The drawing under review shows one solid part. Ordinate dimensions are in mm from its lowest x, y, z. A direction names the side the tool comes from. Round coordinates to 2 decimals unless told otherwise and drop trailing zeros. Write each loop counter-clockwise with the first axis right and the second up, starting at its lowest first coordinate (ties: lowest second). Pieces come first, ordered by that corner, then holes. Notation, with made-up numbers: (82, -34.75) -> (140, -34.75) arc R31 ccw to (140, -0.75) -> close; hole circle Ø1 at (15, 55.25). An arc over 180 degrees is marked (long way). Write item = value, one per line. Start each with the question number.
Item 1: Add section D-D, the plane y = 3.85. State the section outline as (x, z) points, then the cut area to 3 significant figures.
Item 2: Machinability: for the marked faces 1 and 2, which of the approach directions +Z, -Z, +X, -X, +Y, -Y give a long, thin tool a straight path to every point of the face, cutting with its end or side? Answer none if there is none.
Item 3: Add section B-B, the plane y = 0.9. State the section outline as (x, z) points.
Item 4: Add section C-C, the plane z = 4. State the section outline as (x, y) points, then the cut area to 4 significant figures.
Item 5: Add section A-A, the plane x = 20. State the section outline as (y, z) points.
Item 6: Mouldability with a two-part tool opening along Z and no side actions: class the marked faces 3, 4, 5 and 6 as released by +Z, released by -Z, zero draft, split by the parting line, or undercut.
Item 7: To check wall thickness, follow L1, parallel to X at y = 0.7, z = 2.75; L2, parallel to Z at x = 2.75, y = 1.3; L3, parallel to Y at x = 12.25, z = 1.5. State the ranges of each line that lie inside material, in increasing order.
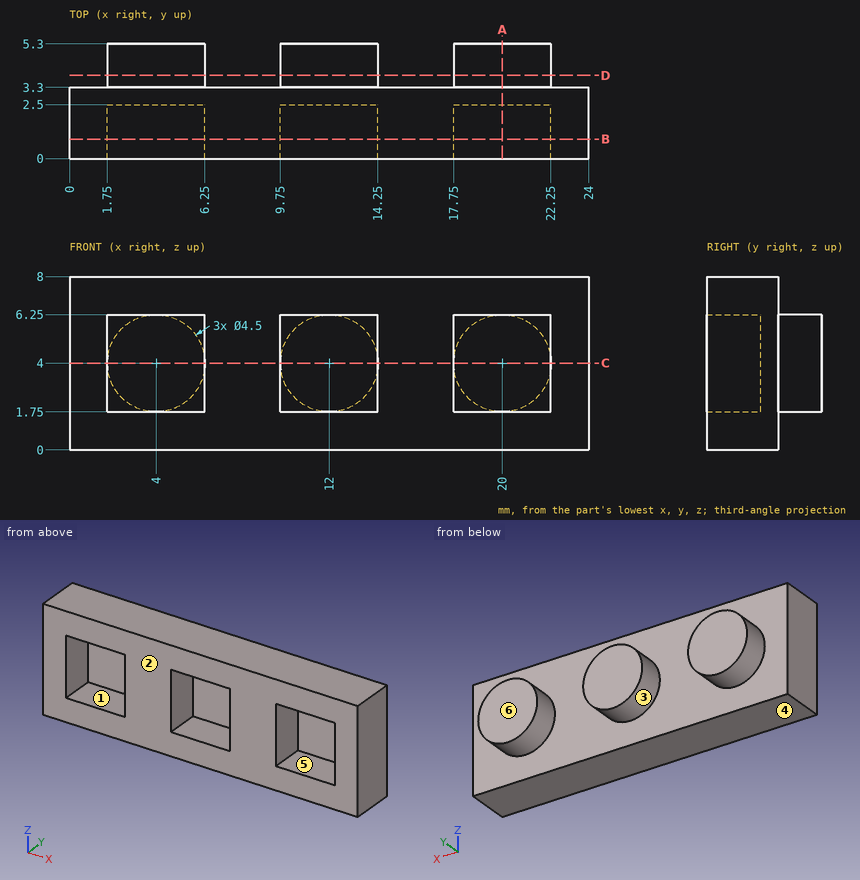
Result set:
q1.outline = circle Ø4.5 at (4, 4); circle Ø4.5 at (12, 4); circle Ø4.5 at (20, 4)
q1.area = 47.7 mm²
q2.face_1 = -Y
q2.face_2 = +Z, -Z, +X, -X, -Y
q3.outline = (0, 0) -> (24, 0) -> (24, 8) -> (0, 8) -> close; hole (1.75, 1.75) -> (6.25, 1.75) -> (6.25, 6.25) -> (1.75, 6.25) -> close; hole (9.75, 1.75) -> (14.25, 1.75) -> (14.25, 6.25) -> (9.75, 6.25) -> close; hole (17.75, 1.75) -> (22.25, 1.75) -> (22.25, 6.25) -> (17.75, 6.25) -> close
q4.outline = (0, 0) -> (1.75, 0) -> (1.75, 2.5) -> (6.25, 2.5) -> (6.25, 0) -> (9.75, 0) -> (9.75, 2.5) -> (14.25, 2.5) -> (14.25, 0) -> (17.75, 0) -> (17.75, 2.5) -> (22.25, 2.5) -> (22.25, 0) -> (24, 0) -> (24, 3.3) -> (22.25, 3.3) -> (22.25, 5.3) -> (17.75, 5.3) -> (17.75, 3.3) -> (14.25, 3.3) -> (14.25, 5.3) -> (9.75, 5.3) -> (9.75, 3.3) -> (6.25, 3.3) -> (6.25, 5.3) -> (1.75, 5.3) -> (1.75, 3.3) -> (0, 3.3) -> close
q4.area = 72.45 mm²
q5.outline = (0, 0) -> (3.3, 0) -> (3.3, 1.75) -> (5.3, 1.75) -> (5.3, 6.25) -> (3.3, 6.25) -> (3.3, 8) -> (0, 8) -> (0, 6.25) -> (2.5, 6.25) -> (2.5, 1.75) -> (0, 1.75) -> close
q6.face_3 = split by the parting line
q6.face_4 = released by -Z
q6.face_5 = undercut
q6.face_6 = zero draft
q7.L1 = 0 to 1.75, 6.25 to 9.75, 14.25 to 17.75, 22.25 to 24
q7.L2 = 0 to 1.75, 6.25 to 8
q7.L3 = 0 to 3.3
